The model under review builds one solid part; all positions refer to its coordinate system, in mm. A direction names the side the tool comes from. Round coordinates to 2 decimals unless told otherwise and drop trailing zeros. Write each loop counter-clockwise with the first axis right and the second up, starting at its lowest first coordinate (ties: lowest second). Pieces come first, ordered by that corner, then holes. Notation, with made-up numbers: (7.25, 44) -> (16.25, 44) arc R28 ccw to (16.25, 81) -> close; hole circle Ø6 at (24, 63.5). An arc over 180 degrees is marked (long way). Answer as a JSON object with one key per item and string values. Group by question number.
1) Mouldability with a two-part tool opening along Z and no side actions: class faces 1 (the cylindrical face through (-67.834, -60.827, 5.112)), 2 (the flat face through (-57, 80, 4)), 3 (the flat face through (-40.75, -73, 5)) as pulls with the +Z half, pulls with the -Z half, needs draft (parallel to the pull), parting line crosses it, or undercut.
2) Insertion check: pin 1 Ø8 at (x, y) = (-47.5, 37) entering from -Z; pin 2 Ø1.6 at (x, y) = (-53, 80) entering from -Z; pin 3 Ø0.9 at (y, z) = (-73, 4) entering from -X. Each pin has a flat end and moves straight along its axis. Give the tip position at first contact, or say it passes through.
3) We need section D-D, the plane y = -8. Write out the cut boundary in (x, z).
4) Machinability: for faces 4 (the flat face through (-72, 85.375, -6)), 5 (the flat face through (-57, 81.375, -1)), 6 (the flat face through (-56.99, 20.88, 26.1)), which of the approach directions +Z, -Z, +X, -X, +Y, -Y give a long, thin tool a straight path to every point of the face, cutting with its end or side? Answer none if there is none.
5) We need section B-B, the plane z = 32. Write out the cut boundary in (x, y), then the cut area to 3 significant figures.
6) We need section C-C, the plane y = 64.5. Write out the cut boundary in (x, z).
7) We need section A-A, the plane x = -63.75. Count the separate pieces of the cut face and the enclosed holes in it, then the cut area to 3 significant figures.
8) To check wall thickness, follow probe 1 along Z at (x, y) = (-66.75, 86.5); probe 2 along X at (y, z) = (83, 16.8); probe 3 along Z at (x, y) = (-70, 31.5). State the ranges of each line that lie inside material, in increasing order. Write a range as [from, to].
from build123d import *

# Parameters (mm, degrees)
SKETCH2_W                = 147.5
SKETCH2_H                = 176.75
BOSS_EXTRUDE1_DEPTH      = 10
SKETCH3_W                = 29
SKETCH3_H                = 15
BOSS_EXTRUDE2_DEPTH      = 34
BOSS_EXTRUDE3_DEPTH      = 34
SKETCH8_W                = 113.5
SKETCH8_H                = 176.75
CUT_EXTRUDE1_DEPTH       = 30
SKETCH9_R                = 2.5
CUT_EXTRUDE2_DEPTH       = 134.016415209
SKETCH10_W               = 3
SKETCH10_H               = 3
CUT_EXTRUDE3_DEPTH       = 3
CUT_EXTRUDE8_DEPTH       = 40
CUT_EXTRUDE8_DEPTH_BACK  = 40
SKETCH11_W               = 10
SKETCH11_H               = 4
SKETCH11_H_2             = 8
SKETCH11_H_3             = 3
SKETCH14_R               = 2.55
CUT_EXTRUDE9_DEPTH       = 40
CUT_EXTRUDE10_DEPTH      = 190.85860157
CUT_EXTRUDE10_DEPTH_BACK = 10
SKETCH15_R               = 1.4
SKETCH16_W               = 12
SKETCH16_H               = 8
CUT_EXTRUDE11_DEPTH      = 116.802867905
FILLET1_R                = 5
SKETCH17_R               = 1.4
CUT_EXTRUDE12_DEPTH      = 10
SKETCH18_R               = 1.4
CUT_EXTRUDE13_DEPTH      = 10
CUT_EXTRUDE14_DEPTH      = 34
FILLET2_R                = 5
SKETCH21_W               = 12
SKETCH21_H               = 10
BOSS_EXTRUDE4_DEPTH      = 5
SKETCH22_W               = 10
SKETCH22_H               = 3
CUT_EXTRUDE15_DEPTH      = 1
SKETCH23_W               = 11
SKETCH23_H               = 3
CUT_EXTRUDE16_DEPTH      = 1
SKETCH24_W               = 32
SKETCH24_H               = 3
CUT_EXTRUDE17_DEPTH      = 1


with BuildPart() as part:
    # Sketch2 → Boss-Extrude1 (new body)
    with BuildSketch(Plane.XY):
        Rectangle(SKETCH2_W, SKETCH2_H)
    extrude(amount=BOSS_EXTRUDE1_DEPTH)

    # Sketch3 → Boss-Extrude2 (add)
    with BuildSketch(Plane.ZY.offset(73.75)):
        with Locations((7.5, 80.875)):
            Rectangle(SKETCH3_W, SKETCH3_H)
        with Locations((7.5, -80.875)):
            Rectangle(SKETCH3_W, SKETCH3_H)
    boss_extrude2 = extrude(amount=-BOSS_EXTRUDE2_DEPTH)

    # Mirror1: Boss-Extrude2 across plane
    add(boss_extrude2.mirror(Plane(origin=(0, 0, 0), x_dir=(0, 0, 1), z_dir=(1, 0, 0))))

    # Sketch5 → Boss-Extrude3 (add)
    with BuildSketch(Plane.ZY.offset(73.75)):
        Polygon((13.717233978, 0), (47.494362324, 23.650999887), (54.37727956, 13.821175356), (66.664560225, 22.424821901), (50.030843571, 46.180231185), (37.743562906, 37.57658464), (41.758597961, 31.84252033), (10, 9.604910635), (10, -9.604910635), (41.758597961, -31.84252033), (37.743562906, -37.57658464), (50.030843571, -46.180231185), (66.664560225, -22.424821901), (54.37727956, -13.821175356), (47.494362324, -23.650999887), align=None)
    extrude(amount=-BOSS_EXTRUDE3_DEPTH)

    # Sketch8 → Cut-Extrude1 (cut)
    with BuildSketch(Plane.XY.offset(22)):
        with Locations((17, 0)):
            Rectangle(SKETCH8_W, SKETCH8_H)
    extrude(amount=-CUT_EXTRUDE1_DEPTH, mode=Mode.SUBTRACT)

    # Sketch9 → Cut-Extrude2 (cut, through all)
    with BuildSketch(Plane(origin=(0, 0, 0), x_dir=(-1, 0, 0), z_dir=(0, 0, -1))):
        with Locations((49.75, 58.375)):
            Circle(SKETCH9_R)
        with Locations((63.75, 58.375)):
            Circle(SKETCH9_R)
        with Locations((49.75, -53.375)):
            Circle(SKETCH9_R)
        with Locations((63.75, -53.375)):
            Circle(SKETCH9_R)
    extrude(amount=-CUT_EXTRUDE2_DEPTH, mode=Mode.SUBTRACT)

    # Sketch10 → Cut-Extrude3 (cut)
    with BuildSketch(Plane(origin=(0, 0, -7), x_dir=(-1, 0, 0), z_dir=(0, 0, -1))):
        with Locations((72.25, 86.875)):
            Rectangle(SKETCH10_W, SKETCH10_H)
    extrude(amount=-CUT_EXTRUDE3_DEPTH, mode=Mode.SUBTRACT)

    # Sketch11 → Cut-Extrude8 (cut, two sides: drawn at the far end of the back side and taken through both)
    with BuildSketch(Plane(origin=(0, 0, 0), x_dir=(-1, 0, 0), z_dir=(0, 0, -1)).offset(-CUT_EXTRUDE8_DEPTH_BACK)):
        with Locations((56.75, -63.375)):
            Rectangle(SKETCH11_W, SKETCH11_H)
        with Locations((56.75, -69.375)):
            Rectangle(SKETCH11_W, SKETCH11_H_2)
        with Locations((56.75, -59.875)):
            Rectangle(SKETCH11_W, SKETCH11_H_3)
        Polygon((42.75, -73.375), (39.75, -73.375), (39.75, -88.375), (73.75, -88.375), (73.75, -73.375), (70.75, -73.375), (61.75, -73.375), (51.75, -73.375), align=None)
    extrude(amount=CUT_EXTRUDE8_DEPTH + CUT_EXTRUDE8_DEPTH_BACK, mode=Mode.SUBTRACT)

    # Sketch14 → Cut-Extrude9 (cut)
    with BuildSketch(Plane.ZY.offset(73.75)):
        with Locations(Location((5, -63.375, 0), (0, 0, 270))):
            Circle(SKETCH14_R)
    extrude(amount=-CUT_EXTRUDE9_DEPTH, mode=Mode.SUBTRACT)

    # Sketch15 → Cut-Extrude10 (cut, two sides: drawn at the far end of the back side and taken through both)
    with BuildSketch(Plane(origin=(0, 88.375, 0), x_dir=(1, 0, 0), z_dir=(0, 1, 0)).offset(-CUT_EXTRUDE10_DEPTH_BACK)):
        with Locations(Location((-46.75, -16.8, 0), (0, 0, 90))):
            Circle(SKETCH15_R)
        with Locations(Location((-66.75, -16.8, 0), (0, 0, 90))):
            Circle(SKETCH15_R)
        with Locations(Location((-66.75, -0.8, 0), (0, 0, 90))):
            Circle(SKETCH15_R)
        with Locations(Location((-46.75, -0.8, 0), (0, 0, 90))):
            Circle(SKETCH15_R)
    extrude(amount=CUT_EXTRUDE10_DEPTH + CUT_EXTRUDE10_DEPTH_BACK, mode=Mode.SUBTRACT)

    # Sketch16 → Cut-Extrude11 (cut, through all)
    with BuildSketch(Plane.ZY.offset(73.75)):
        Polygon((-7, 73.375), (0, 73.375), (4, 73.375), (4, 81.375), (-7, 81.375), (-7, 79.375), align=None)
        with Locations((16, 77.375)):
            Rectangle(SKETCH16_W, SKETCH16_H)
    extrude(amount=-CUT_EXTRUDE11_DEPTH, mode=Mode.SUBTRACT)

    # Fillet1
    # the kernel refuses this fillet: 5 mm, written as the material it adds along each edge
    with BuildSketch(Plane(origin=(-73.75, 73.375, 4), x_dir=(0, 1, 0), z_dir=(1, 0, 0))) as fillet1_piece_1:
        with BuildLine():
            CenterArc((4.898979486, -5), FILLET1_R, 90, 78.463040967)
            Line((0, -4), (-0.09797959, -3.98))
            ThreePointArc((-0.09797959, -3.98), (-0.1, -2), (-0.1, 0))
            Line((-0.1, 0), (0, 0.1))
            Line((0, 0.1), (4.898979486, 0.1))
            Line((4.898979486, 0.1), (4.898979486, 0))
        make_face()
    extrude(amount=34)

    # Sketch17 → Cut-Extrude12 (cut)
    with BuildSketch(Plane(origin=(0, 38.699638206, 55.268811165), x_dir=(1, 0, 0), z_dir=(0, 0.5735764363510447, 0.8191520442889927))):
        with Locations(Location((-66.75, 3.932117818, 0), (0, 0, 270))):
            Circle(SKETCH17_R)
        with Locations(Location((-46.75, 3.932117818, 0), (0, 0, 270))):
            Circle(SKETCH17_R)
        with Locations(Location((-46.75, -12.067882182, 0), (0, 0, 270))):
            Circle(SKETCH17_R)
        with Locations(Location((-66.75, -12.067882182, 0), (0, 0, 270))):
            Circle(SKETCH17_R)
    extrude(amount=-CUT_EXTRUDE12_DEPTH, mode=Mode.SUBTRACT)

    # Sketch18 → Cut-Extrude13 (cut)
    with BuildSketch(Plane(origin=(0, -38.699638206, 55.268811165), x_dir=(1, 0, 0), z_dir=(0, -0.5735764363510447, 0.8191520442889929))):
        with Locations(Location((-46.75, -3.932117818, 0), (0, 0, 270))):
            Circle(SKETCH18_R)
        with Locations(Location((-66.75, -3.932117818, 0), (0, 0, 270))):
            Circle(SKETCH18_R)
        with Locations(Location((-66.75, 12.067882182, 0), (0, 0, 270))):
            Circle(SKETCH18_R)
        with Locations(Location((-46.75, 12.067882182, 0), (0, 0, 270))):
            Circle(SKETCH18_R)
    extrude(amount=-CUT_EXTRUDE13_DEPTH, mode=Mode.SUBTRACT)

    # Sketch20 → Cut-Extrude14 (cut)
    with BuildSketch(Plane.ZY.offset(73.75)):
        Polygon((37.743562906, 37.57658464), (41.758597961, 31.84252033), (44.052903706, 28.565912153), (50.60612006, 33.154523644), (44.296779261, 42.165196131), align=None)
        Polygon((47.494362324, 23.650999887), (54.37727956, 13.821175356), (60.930495915, 18.409786846), (54.047578679, 28.239611378), align=None)
        Polygon((54.047578679, -28.239611378), (47.494362324, -23.650999887), (54.37727956, -13.821175356), (60.930495915, -18.409786846), align=None)
        Polygon((50.60612006, -33.154523644), (44.052903706, -28.565912153), (41.758597961, -31.84252033), (37.743562906, -37.57658464), (44.296779261, -42.165196131), align=None)
    extrude(amount=-CUT_EXTRUDE14_DEPTH, mode=Mode.SUBTRACT)

    # Fillet2
    # the kernel refuses this fillet: 5 mm, written as the material it adds along each edge
    with BuildSketch(Plane(origin=(-73.75, -28.565912153, 44.052903706), x_dir=(0, -0.573576436351048, 0.8191520442889905), z_dir=(1, 0, 0))) as fillet2_piece_1:
        with BuildLine():
            CenterArc((4.898979486, 5), FILLET2_R, 191.536959033, 78.463040967)
            Line((0, 4), (-0.09797959, 3.98))
            ThreePointArc((-0.09797959, 3.98), (-0.1, 2), (-0.1, 0))
            Line((-0.1, 0), (0, -0.1))
            Line((0, -0.1), (4.898979486, -0.1))
            Line((4.898979486, -0.1), (4.898979486, 0))
        make_face()
    extrude(amount=34)
    with BuildSketch(Plane(origin=(-73.75, 28.565912153, 44.052903706), x_dir=(0, 0.8191520442898972, -0.5735764363497533), z_dir=(1, 0, 0))) as fillet2_piece_2:
        with BuildLine():
            CenterArc((5, 4.898979486), FILLET2_R, 180, 78.463040967)
            Line((0, 4.898979486), (-0.1, 4.898979486))
            Line((-0.1, 4.898979486), (-0.1, 0))
            Line((-0.1, 0), (0, -0.1))
            ThreePointArc((0, -0.1), (2, -0.1), (3.98, -0.09797959))
            Line((3.98, -0.09797959), (4, 0))
        make_face()
    extrude(amount=34)

    # Sketch21 → Boss-Extrude4 (add)
    with BuildSketch(Plane.XZ.offset(73.375)):
        with Locations((-67.75, 5)):
            Rectangle(SKETCH21_W, SKETCH21_H)
        with Locations((-45.75, 5)):
            Rectangle(SKETCH21_W, SKETCH21_H)
    extrude(amount=BOSS_EXTRUDE4_DEPTH)

    # Sketch22 → Cut-Extrude15 (cut)
    with BuildSketch(Plane.ZY.offset(73.75)):
        with Locations((5, -72.875)):
            Rectangle(SKETCH22_W, SKETCH22_H)
    cut_extrude15 = extrude(amount=-CUT_EXTRUDE15_DEPTH, mode=Mode.SUBTRACT)

    # Mirror2: Cut-Extrude15 across plane
    add(cut_extrude15.mirror(Plane.ZY.offset(56.75)), mode=Mode.SUBTRACT)

    # Sketch23 → Cut-Extrude16 (cut)
    with BuildSketch(Plane(origin=(0, 0, 0), x_dir=(-1, 0, 0), z_dir=(0, 0, -1))):
        with Locations((67.25, -72.875)):
            Rectangle(SKETCH23_W, SKETCH23_H)
        with Locations((46.25, -72.875)):
            Rectangle(SKETCH23_W, SKETCH23_H)
    extrude(amount=-CUT_EXTRUDE16_DEPTH, mode=Mode.SUBTRACT)

    # Sketch24 → Cut-Extrude17 (cut)
    with BuildSketch(Plane.XY.offset(10)):
        with Locations((-56.75, -72.875)):
            Rectangle(SKETCH24_W, SKETCH24_H)
    extrude(amount=-CUT_EXTRUDE17_DEPTH, mode=Mode.SUBTRACT)


solid = part.part
Here are the results:
{
 "1": {"face 1": "undercut", "face 2": "pulls with the -Z half", "face 3": "needs draft"},
 "2": {"pin 1": "stops at z = 0", "pin 2": "stops at z = 4", "pin 3": "stops at x = -72.75"},
 "3": {"outline": "(-73.75, 0) -> (-39.75, 0) -> (-39.75, 25.14) -> (-73.75, 25.14) -> close"},
 "4": {"face 4": "-Z, -X, +Y", "face 5": "-Z, +X, -X", "face 6": "+X, -X"},
 "5": {"outline": "(-73.75, -25.01) -> (-39.75, -25.01) -> (-39.75, -12.8) -> (-73.75, -12.8) -> close; (-73.75, 12.8) -> (-39.75, 12.8) -> (-39.75, 25.01) -> (-73.75, 25.01) -> close", "area": "830 mm^2"},
 "6": {"outline": "(-73.75, 0) -> (-39.75, 0) -> (-39.75, 10) -> (-73.75, 10) -> close"},
 "7": {"separate pieces": "3", "enclosed holes": "1", "area": "2,990 mm^2"},
 "8": {"probe 1": "z = [-7, -0.6], [2.2, 15.4], [18.2, 22]", "probe 2": "x = [-73.75, -68.15], [-65.35, -48.15], [-45.35, -39.75]", "probe 3": "z = [0, 10], [41.27, 42.16], [48.24, 60.31]"}
}
